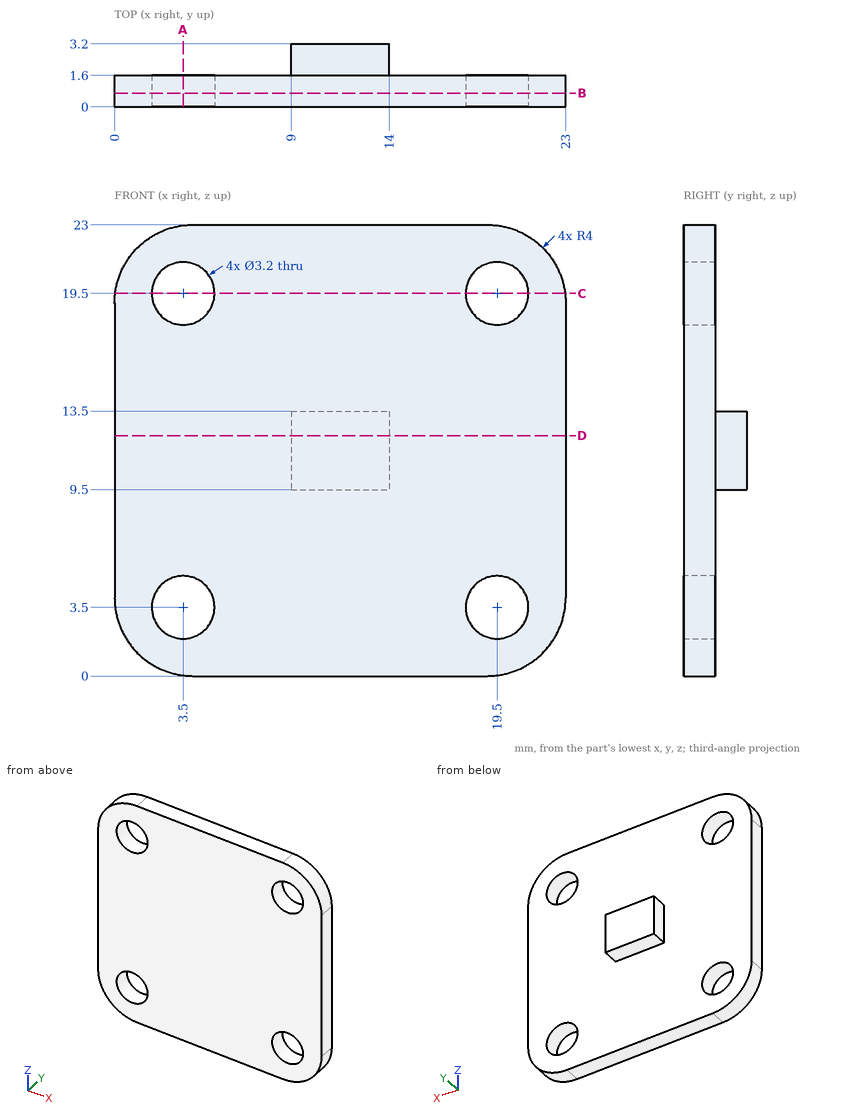
Study the drawing (mm; zero at the part's minimum x, y, z) and answer. Coordinates: 2 decimals unless noted, no trailing zeros. Write each loop counter-clockwise with the first axis right and the second up, starting at its lowest first coordinate (ties: lowest second). Pieces come first, ordered by that corner, then holes. Notation, with made-up numbers: (4, 88.25) -> (19, 88.25) arc R12 ccw to (19, 95.25) -> close; hole circle Ø7 at (82.25, 62). An arc over 180 degrees is marked (long way). Write each question's results on one line, items separated by ' | '. Start each with the question number.
1) A cutting plane is placed at B-B (y = 0.7). Determine the outline of the cut face in (x, z).
2) A cutting plane is placed at D-D (z = 12.25). Determine the outline of the cut face in (x, y), then the cut area to 3 significant figures.
3) Straight lines are drawn through the part: probe 1 along X at (y, z) = (1.1, 3.5); probe 2 along X at (y, z) = (0.2, 4.25); probe 3 along Z at (x, y) = (13.75, 2.1). For each, find the intervals that lie inside material, in ascending order.
4) A cutting plane is placed at C-C (z = 19.5). Determine the outline of the cut face in (x, y), then the cut area to 3 significant figures.
5) A cutting plane is placed at A-A (x = 3.5). Determine the outline of the cut face in (y, z), then the cut area to 3 significant figures.
6) Flat-ended cylindrical pins translate along their axes: pin 1 Ø8 at (x, z) = (3, 10) entering from +Y; pin 2 Ø12 at (x, z) = (15.5, 5.5) entering from -Y; pin 3 Ø1.9 at (x, z) = (19.5, 19.5) entering from +Y; pin 4 Ø0.5 at (x, y) = (12.5, 2.5) entering from -Z. Find the tip coordinate at first contact, or state that the pin passes through.
Values follow:
1) outline: (0, 4) arc R4 ccw to (4, 0) -> (19, 0) arc R4 ccw to (23, 4) -> (23, 19) arc R4 ccw to (19, 23) -> (4, 23) arc R4 ccw to (0, 19) -> close; hole circle Ø3.2 at (3.5, 3.5); hole circle Ø3.2 at (3.5, 19.5); hole circle Ø3.2 at (19.5, 3.5); hole circle Ø3.2 at (19.5, 19.5)
2) outline: (0, 0) -> (23, 0) -> (23, 1.6) -> (14, 1.6) -> (14, 3.2) -> (9, 3.2) -> (9, 1.6) -> (0, 1.6) -> close | area: 44.8 mm²
3) probe 1: 0.03 to 1.9, 5.1 to 17.9, 21.1 to 22.97 | probe 2: 0 to 2.09, 4.91 to 18.09, 20.91 to 23 | probe 3: 9.5 to 13.5
4) outline: (0.03, 0) -> (1.9, 0) -> (1.9, 1.6) -> (0.03, 1.6) -> close; (5.1, 0) -> (17.9, 0) -> (17.9, 1.6) -> (5.1, 1.6) -> close; (21.1, 0) -> (22.97, 0) -> (22.97, 1.6) -> (21.1, 1.6) -> close | area: 26.5 mm²
5) outline: (0, 0.03) -> (1.6, 0.03) -> (1.6, 1.9) -> (0, 1.9) -> close; (0, 5.1) -> (1.6, 5.1) -> (1.6, 17.9) -> (0, 17.9) -> close; (0, 21.1) -> (1.6, 21.1) -> (1.6, 22.97) -> (0, 22.97) -> close | area: 26.5 mm²
6) pin 1: y = 1.6 | pin 2: y = 0 | pin 3: through | pin 4: z = 9.5
